Read the model definition and answer for the solid it produces. Units are mm, in the model's axes. A direction names the side the tool comes from. Coordinates: 2 decimals unless noted, no trailing zeros. Write each loop counter-clockwise with the first axis right and the second up, starting at its lowest first coordinate (ties: lowest second). Pieces come first, ordered by that corner, then holes.
(1) Section C-C on z = -4.25 is taken. Write down the section's boundary in (x, y), then the cut area to 3 significant figures.
(2) Which of the six approach directions +Z, -Z, +X, -X, +Y, -Y give full straight-line access (tool end or side, diameter ignored) to faces 1 (the cylindrical face through (-6.98, 2.2, -4.93)), 2 (the cylindrical face through (7.12, 7.02, 1.97)), 3 (the flat face through (6, 0, 4))?
(3) Find the intervals of material crossed by probe 1 along Y at (x, z) = (-18, 2.75); probe 2 along Y at (x, z) = (0, -1); probe 3 along X at (y, z) = (16.5, 3), in increasing order.
(4) Given pin 1 (3 mm diameter, centred on x = -13.5, z = 1.5, fed in from -Y); pin 2 (1.2 mm diameter, centred on x = 19.5, z = 2, fed in from +Y); pin 3 (4.5 mm diameter, centred on x = 17, z = 2.5, fed in from -Y), each flat-ended and moving along its own axis, determine where each tip first touches the part or whether it passes through.
(5) Section D-D on x = -21 is taken. State how many separate pieces and enclosed holes the cut face has, then the cut area to 3 significant figures.
(6) Section A-A on y = 0 is taken. Write down the section's boundary in (x, z).
(7) Section B-B on x = 0 is taken. Write down the section's boundary in (y, z), then the cut area to 3 significant figures.
(8) The mould has two halves that part along Y. Classify faces 4 (the cylindrical face through (-29.97, 1.32, 0.2)), 5 (the cylindrical face through (16.81, 17.13, 1.97)), 6 (the flat face through (-3, -17, 2)), 7 (the flat face through (6, -6, 0)): +Y half, -Y half, draft (parallel to the pull), parting line (faces both ways), or undercut.
from build123d import *

# Parameters (mm, degrees)
CROQUIS1_R              = 30
SALIENTE_EXTRUIR1_DEPTH = 4
CROQUIS4_R              = 7.319391613
SALIENTE_EXTRUIR2_DEPTH = 10
CORTAR_EXTRUIR1_DEPTH   = 10
CORTAR_EXTRUIR2_DEPTH   = 15


with BuildPart() as part:
    # Croquis1 → Saliente-Extruir1 (new body)
    with BuildSketch(Plane.XY):
        Circle(CROQUIS1_R)
    extrude(amount=SALIENTE_EXTRUIR1_DEPTH)

    # Croquis3 → Cortar-Revolución1 (revolve, cut)
    with BuildSketch(Plane(origin=(0, 0, 0), x_dir=(1, 0, 0), z_dir=(0, 1, 0))):
        Polygon((-30, -4), (-30, -3.587135196), (-28.759048166, -2), (-30, -0.412864804), (-30, 0), (-32.403502023, 0), (-32.403502023, -4), align=None)
    revolve(axis=Axis((0, 0, -0.500745856), (0, 0, 1)), mode=Mode.SUBTRACT)

    # Croquis4 → Saliente-Extruir2 (add)
    with BuildSketch(Plane(origin=(0, 0, 0), x_dir=(-1, 0, 0), z_dir=(0, 0, -1))):
        Circle(CROQUIS4_R)
    extrude(amount=SALIENTE_EXTRUIR2_DEPTH)

    # Croquis5 → Cortar-Extruir1 (cut)
    with BuildSketch(Plane(origin=(0, 0, 0), x_dir=(-1, 0, 0), z_dir=(0, 0, -1))):
        with BuildLine():
            Line((-23.8117618, -3), (-9.539392014, -3))
            ThreePointArc((-9.539392014, -3), (-7.071067812, -7.071067812), (-3, -9.539392014))
            Line((-3, -9.539392014), (-3, -23.8117618))
            ThreePointArc((-3, -23.8117618), (-16.970562748, -16.970562748), (-23.8117618, -3))
        make_face()
        with BuildLine():
            Line((-23.8117618, 3), (-9.539392014, 3))
            ThreePointArc((-9.539392014, 3), (-7.071067812, 7.071067812), (-3, 9.539392014))
            Line((-3, 9.539392014), (-3, 23.8117618))
            ThreePointArc((-3, 23.8117618), (-16.970562748, 16.970562748), (-23.8117618, 3))
        make_face()
        with BuildLine():
            Line((3, 23.8117618), (3, 9.539392014))
            ThreePointArc((3, 9.539392014), (7.071067812, 7.071067812), (9.539392014, 3))
            Line((9.539392014, 3), (23.8117618, 3))
            ThreePointArc((23.8117618, 3), (16.970562748, 16.970562748), (3, 23.8117618))
        make_face()
        with BuildLine():
            Line((23.8117618, -3), (9.539392014, -3))
            ThreePointArc((9.539392014, -3), (7.071067812, -7.071067812), (3, -9.539392014))
            Line((3, -9.539392014), (3, -23.8117618))
            ThreePointArc((3, -23.8117618), (16.970562748, -16.970562748), (23.8117618, -3))
        make_face()
    extrude(amount=-CORTAR_EXTRUIR1_DEPTH, mode=Mode.SUBTRACT)

    # Croquis6 → Cortar-Extruir2 (cut, through all)
    with BuildSketch(Plane(origin=(0, 0, -10), x_dir=(-1, 0, 0), z_dir=(0, 0, -1))):
        with BuildLine():
            Line((1.5, -2.123676058), (-1.5, -2.123676058))
            ThreePointArc((-1.5, -2.123676058), (0, 2.6), (1.5, -2.123676058))
        make_face()
    extrude(amount=-CORTAR_EXTRUIR2_DEPTH, mode=Mode.SUBTRACT)


solid = part.part
Response:
1. outline: circle Ø14.64 at (0, 0); hole (-1.5, -2.12) - (1.5, -2.12) arc R2.6 ccw (long way) to start
1. area: 148 mm2
2. face 1: -Z
2. face 2: +Z, -Z
2. face 3: +Z, +X, -X, +Y, -Y
3. probe 1: y = -23.18 to -15.87, -3 to 3, 15.87 to 23.18
3. probe 2: y = -7.32 to -2.12, 2.6 to 7.32
3. probe 3: x = -24.5 to -17.43, -3 to 3, 17.43 to 24.5
4. pin 1: stops at y = -27.29
4. pin 2: stops at y = 21.97
4. pin 3: stops at y = -25.96
5. separate pieces: 3
5. enclosed holes: 0
5. area: 96.8 mm2
6. outline: (-30, 0) - (-7.32, 0) - (-7.32, -10) - (-2.6, -10) - (-2.6, 4) - (-30, 4) - (-30, 3.59) - (-28.76, 2) - (-30, 0.41) - close; (2.6, -10) - (7.32, -10) - (7.32, 0) - (30, 0) - (30, 0.41) - (28.76, 2) - (30, 3.59) - (30, 4) - (2.6, 4) - close
7. outline: (-30, 0) - (-7.32, 0) - (-7.32, -10) - (-2.12, -10) - (-2.12, 4) - (-30, 4) - (-30, 3.59) - (-28.76, 2) - (-30, 0.41) - close; (2.6, -10) - (7.32, -10) - (7.32, 0) - (30, 0) - (30, 0.41) - (28.76, 2) - (30, 3.59) - (30, 4) - (2.6, 4) - close
7. area: 316 mm2
8. face 4: parting line
8. face 5: undercut
8. face 6: undercut
8. face 7: draft
